Could you check a few things on this model? Use its own coordinates, in mm. Give positions to 0.01 mm unless a question says otherwise; leave off trailing zeros. Write each loop counter-clockwise with the first axis right and the second up, starting at its lowest first coordinate (ties: lowest second). Pieces come first, ordered by that corner, then holes. Notation, with made-up numbers: M -36,68.25 L 1,68.25 A15 cw 1,92.25 Z; hole C 33.5,74.25 d2. An arc over 180 degrees is marked long. One line per item, written item: value.
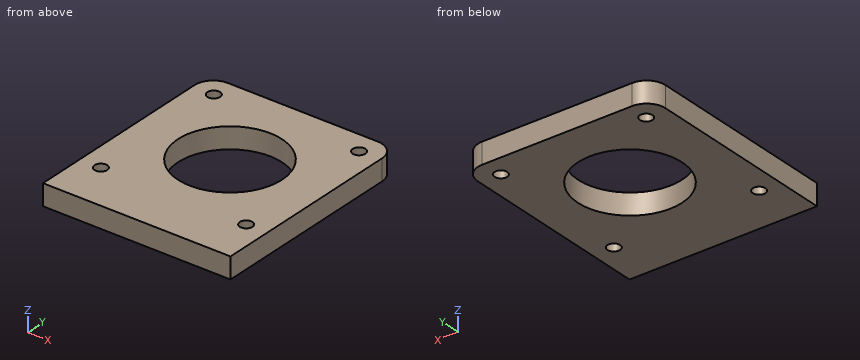
```python
from build123d import *

# Parameters (mm, degrees)
SKETCH1_W           = 40
SKETCH1_H           = 45.6
SKETCH1_R           = 1.35
SKETCH1_R_2         = 11.1
BOSS_EXTRUDE1_DEPTH = 4.5
FILLET1_R           = 4


with BuildPart() as part:
    # Sketch1 → Boss-Extrude1 (new body)
    with BuildSketch(Plane.XY):
        with Locations((0, -2.8)):
            Rectangle(SKETCH1_W, SKETCH1_H)
        with Locations((-15.5, -15.5)):
            Circle(SKETCH1_R, mode=Mode.SUBTRACT)
        with Locations((15.5, -15.5)):
            Circle(SKETCH1_R, mode=Mode.SUBTRACT)
        Circle(SKETCH1_R_2, mode=Mode.SUBTRACT)
        with Locations((-15.5, 15.5)):
            Circle(SKETCH1_R, mode=Mode.SUBTRACT)
        with Locations((15.5, 15.5)):
            Circle(SKETCH1_R, mode=Mode.SUBTRACT)
    extrude(amount=BOSS_EXTRUDE1_DEPTH)

    # Fillet1
    fillet1_edges = [part.edges().sort_by_distance(p)[0] for p in [
        (-20, 20, 2.25),
        (20, 20, 2.25),
    ]]
    fillet(fillet1_edges, radius=FILLET1_R)


solid = part.part
```
1) If we section it at C-C, the plane x = -15.5: Write out the boundary of the cut face in (y, z).
Outcome:
outline: M -25.6,0 L -16.85,0 L -16.85,4.5 L -25.6,4.5 Z; M -14.15,0 L 14.15,0 L 14.15,4.5 L -14.15,4.5 Z; M 16.85,0 L 20,0 L 20,4.5 L 16.85,4.5 Z
2) If we section it at D-D, the plane y = 0: Write out the boundary of the cut face in (x, z), then the cut area to 3 significant figures.
Outcome:
outline: M -20,0 L -11.1,0 L -11.1,4.5 L -20,4.5 Z; M 11.1,0 L 20,0 L 20,4.5 L 11.1,4.5 Z
area: 80.1 mm^2
3) Please list where these lines run through material, in increasing order: L1, parallel to Y at x = -15.5, z = 2.5; L2, parallel to X at y = -15, z = 3.55; L3, parallel to Y at x = 0, z = 1.65. Write a range as from..to.
Outcome:
L1: y = -25.6..-16.85, -14.15..14.15, 16.85..20
L2: x = -20..-16.75, -14.25..14.25, 16.75..20
L3: y = -25.6..-11.1, 11.1..20
4) If we section it at A-A, the plane x = 0: Write out the boundary of the cut face in (y, z).
Outcome:
outline: M -25.6,0 L -11.1,0 L -11.1,4.5 L -25.6,4.5 Z; M 11.1,0 L 20,0 L 20,4.5 L 11.1,4.5 Z
5) If we section it at B-B, the plane y = 15.5: Write out the boundary of the cut face in (x, z), then the cut area to 3 significant figures.
Outcome:
outline: M -20,0 L -16.85,0 L -16.85,4.5 L -20,4.5 Z; M -14.15,0 L 14.15,0 L 14.15,4.5 L -14.15,4.5 Z; M 16.85,0 L 20,0 L 20,4.5 L 16.85,4.5 Z
area: 156 mm^2
6) I'm going to push a flat-ended pin straight in: pin 1 (2.5 mm diameter, centred on x = 15.5, y = -15.5, fed in from +Z) (3 decimals). Where does the tip first touch, or does it pass through?
Outcome:
pin 1: passes through
